Geometry check sheet. Reference: the model listing, model coordinates, mm. Face numbers are marked on the shaded views. A direction names the side the tool comes from. Give positions to 0.01 mm unless a question says otherwise; leave off trailing zeros. Write each loop counter-clockwise with the first axis right and the second up, starting at its lowest first coordinate (ties: lowest second). Pieces come first, ordered by that corner, then holes. Notation, with made-up numbers: M -29.5,29.5 L -4.5,29.5 A13 cw -4.5,34.5 Z; hole C 16.5,-12 d1. An arc over 180 degrees is marked long. Use one line per item in the form item = value. Start each with the question number.
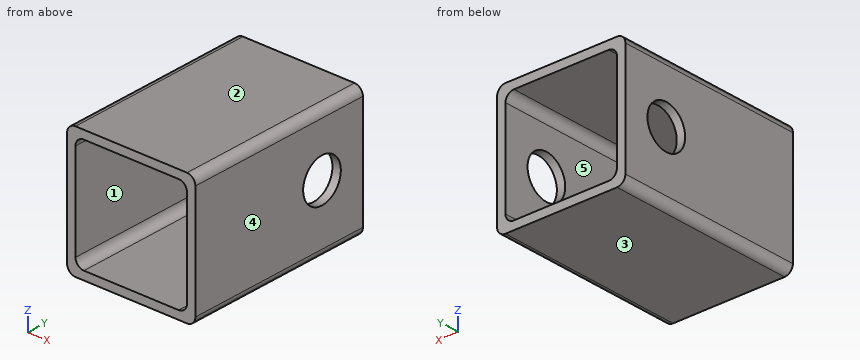
```python
from build123d import *

# Parameters (mm, degrees)
SQUARE_TUBE_75X049_1_DEPTH = 28.221723784
SKETCH3_R                  = 3.175
CUT_EXTRUDE1_DEPTH         = 36.356665826


with BuildPart() as part:
    # Sketch1 → Square tube 75X049(1) (new body)
    with BuildSketch(Plane(origin=(0, 28.221723784, 0), x_dir=(0, 0, -1), z_dir=(0, -1, 0))):
        with BuildLine():
            Line((-8.2804, 9.525), (8.2804, 9.525))
            ThreePointArc((8.2804, 9.525), (9.1604651, 9.1604651), (9.525, 8.2804))
            Line((9.525, 8.2804), (9.525, -8.2804))
            ThreePointArc((9.525, -8.2804), (9.1604651, -9.1604651), (8.2804, -9.525))
            Line((8.2804, -9.525), (-8.2804, -9.525))
            ThreePointArc((-8.2804, -9.525), (-9.1604651, -9.1604651), (-9.525, -8.2804))
            Line((-9.525, -8.2804), (-9.525, 8.2804))
            ThreePointArc((-9.525, 8.2804), (-9.1604651, 9.1604651), (-8.2804, 9.525))
        make_face()
        with BuildLine():
            Line((-8.2804, 7.0358), (-8.2804, -7.0358))
            ThreePointArc((-8.2804, -7.0358), (-7.9158651, -7.9158651), (-7.0358, -8.2804))
            Line((-7.0358, -8.2804), (7.0358, -8.2804))
            ThreePointArc((7.0358, -8.2804), (7.9158651, -7.9158651), (8.2804, -7.0358))
            Line((8.2804, -7.0358), (8.2804, 7.0358))
            ThreePointArc((8.2804, 7.0358), (7.9158651, 7.9158651), (7.0358, 8.2804))
            Line((7.0358, 8.2804), (-7.0358, 8.2804))
            ThreePointArc((-7.0358, 8.2804), (-7.9158651, 7.9158651), (-8.2804, 7.0358))
        make_face(mode=Mode.SUBTRACT)
    extrude(amount=SQUARE_TUBE_75X049_1_DEPTH)

    # Sketch3 → Cut-Extrude1 (cut, through all)
    with BuildSketch(Plane(origin=(9.525, 0, 0), x_dir=(0, 0, -1), z_dir=(1, 0, 0))):
        with Locations((-0.431467727, 21.331601206)):
            Circle(SKETCH3_R)
    extrude(amount=-CUT_EXTRUDE1_DEPTH, mode=Mode.SUBTRACT)


solid = part.part
```
(1) Depth check by flat-ended pin: pin 1 (5 mm diameter, centred on x = -4, z = -3.5, fed in from +Y). Enter the tip coordinate at first touch or a pass-through.
(2) Tool access check on the marked faces 4 and 5. Record the directions out of +Z, -Z, +X, -X, +Y, -Y that give a thin tool (end or side, any length) a straight path to the whole face; none if there is none.
(3) Thickness scan on probe 1 along Z at (x, y) = (6.25, 26.75) (3 decimals); probe 2 along X at (y, z) = (14.5, -7.5) (3 decimals). Record the ranges inside material, lowest first. Write a range as [from, to].
(4) Sectioned sample at C-C, the plane z = -3.25. Record the boundary of the cut face in (x, y) (3 decimals), plus the area to 3 significant figures.
(5) Draft check along Z on the marked faces 1, 2 and 3. Enter one of: released by +Z, released by -Z, zero draft, split by the parting line, or undercut.
(6) Sectioned sample at B-B, the plane y = 14.5. Record the boundary of the cut face in (x, z) (3 decimals).
(7) Sectioned sample at A-A, the plane x = -2. Record the boundary of the cut face in (y, z) (3 decimals).
(8) Sectioned sample at D-D, the plane z = 1. Record the boundary of the cut face in (x, y) (3 decimals), plus the area to 3 significant figures.
Numbers:
q1.pin_1 = through
q2.face_4 = +Z, -Z, +X, +Y, -Y
q2.face_5 = +Y, -Y
q3.probe_1 = [-9.525, -8.28], [8.28, 9.525]
q3.probe_2 = [-9.525, -8.191], [8.191, 9.525]
q4.outline = M -9.525,0 L -8.28,0 L -8.28,28.222 L -9.525,28.222 Z; M 8.28,0 L 9.525,0 L 9.525,28.222 L 8.28,28.222 Z
q4.area = 70.2 mm2
q5.face_1 = undercut
q5.face_2 = released by +Z
q5.face_3 = released by -Z
q6.outline = M -9.525,-8.28 A1.245 ccw -8.28,-9.525 L 8.28,-9.525 A1.245 ccw 9.525,-8.28 L 9.525,8.28 A1.245 ccw 8.28,9.525 L -8.28,9.525 A1.245 ccw -9.525,8.28 Z; hole M -8.28,-7.036 A1.245 ccw -7.036,-8.28 L 7.036,-8.28 A1.245 ccw 8.28,-7.036 L 8.28,7.036 A1.245 ccw 7.036,8.28 L -7.036,8.28 A1.245 ccw -8.28,7.036 Z
q7.outline = M 0,-9.525 L 28.222,-9.525 L 28.222,-8.28 L 0,-8.28 Z; M 0,8.28 L 28.222,8.28 L 28.222,9.525 L 0,9.525 Z
q8.outline = M -9.525,0 L -8.28,0 L -8.28,18.208 L -9.525,18.208 Z; M -9.525,24.455 L -8.28,24.455 L -8.28,28.222 L -9.525,28.222 Z; M 8.28,0 L 9.525,0 L 9.525,18.208 L 8.28,18.208 Z; M 8.28,24.455 L 9.525,24.455 L 9.525,28.222 L 8.28,28.222 Z
q8.area = 54.7 mm2
